Design review of the part built by this model. Coordinates are the model's own, in mm. A direction names the side the tool comes from. Coordinates: 2 decimals unless noted, no trailing zeros. Loops run counter-clockwise (first coordinate to the right, second up) from the corner with the lowest first, then second, coordinate; pieces in that order, holes last.
Q1. Wall thickness on probe 1 along Y at (x, z) = (-2.4, 0.15); probe 2 along X at (y, z) = (-8.5, -0.4); probe 3 along Z at (x, y) = (1.35, -14.25): over which ranges is each line inside the solid? List them lowest first.
Q2. Add section A-A on z = 0. Give the boundary of the cut face in (x, y).
Q3. For P1, Ø3, axis at x = 1, y = -8.5, coming from the -Z side; P2, Ø1, axis at x = 0, y = -5, coming from the +Z side; P3, Ø1.2, axis at x = 0, z = 0, coming from the +Y side, all flat-tipped, find the tip position at first contact; note any pin that passes through.
Q4. Draft analysis for pull direction Z (two halves, no side actions). For faces 3 (the face through (0, -2, 0)), 4 (the face through (0.63, -0.99, -1.08)), 5 (the face through (1.5, -8.92, -0.07)), 6 (the face through (2, -3, 0)), state which applies: released by +Z, released by -Z, zero draft, split by the parting line, or undercut.
Q5. Add section B-B on y = -5.75. Give the boundary of the cut face in (x, z).
Q6. Machinability: for faces 1 (the face through (0.616, -0.987, 1.088)), 2 (the face through (0.596, -1.58, 2.685)), which of the approach directions +Z, -Z, +X, -X, +Y, -Y give a long, thin tool a straight path to every point of the face, cutting with its end or side? Answer none if there is none.
```python
from build123d import *

# Parameters (mm, degrees)
CHAMFER1_SIZE      = 0.25
FILLET1_R          = 0.2
CUT_EXTRUDE1_DEPTH = 2
FILLET2_R          = 0.1


with BuildPart() as part:
    # Sketch1 → Revolve1 (revolve)
    with BuildSketch(Plane.XY):
        Polygon((0, -15), (-1.5, -15), (-1.5, -3), (-2.75, -3), (-2.75, 0), (0, 0), align=None)
    revolve(axis=Axis((0, 0, 0), (0, -1, 0)))

    # Chamfer1
    chamfer1_edges = [part.edges().sort_by_distance(p)[0] for p in [
        (1.5, -3, 0),
        (1.5, -15, 0),
    ]]
    chamfer(chamfer1_edges, length=CHAMFER1_SIZE)

    # Fillet1
    fillet1_edges = [part.edges().sort_by_distance(p)[0] for p in [
        (2.75, 0, 0),
    ]]
    fillet(fillet1_edges, radius=FILLET1_R)

    # Sketch2 → Cut-Extrude1 (cut)
    with BuildSketch(Plane(origin=(0, 0, 0), x_dir=(1, 0, 0), z_dir=(0, 1, 0))):
        Polygon((0, 1.443375673), (-1.25, 0.721687836), (-1.25, -0.721687836), (0, -1.443375673), (1.25, -0.721687836), (1.25, 0.721687836), align=None)
    extrude(amount=-CUT_EXTRUDE1_DEPTH, mode=Mode.SUBTRACT)

    # Fillet2
    fillet2_edges = [part.edges().sort_by_distance(p)[0] for p in [
        (0.625, -2, -1.082531755),
        (1.25, -2, 0),
        (0.625, -2, 1.082531755),
        (-0.625, -2, 1.082531755),
        (-1.25, -2, 0),
        (-0.625, -2, -1.082531755),
        (0.625, 0, -1.082531755),
        (-0.625, 0, -1.082531755),
        (-1.25, 0, 0),
        (-0.625, 0, 1.082531755),
        (0.625, 0, 1.082531755),
        (1.25, 0, 0),
    ]]
    fillet(fillet2_edges, radius=FILLET2_R)


solid = part.part
```
Entries:
1. probe 1: y = -3 to 0
1. probe 2: x = -1.45 to 1.45
1. probe 3: z = -0.65 to 0.65
2. outline: (-2.75, -3) - (-1.75, -3) - (-1.5, -3.25) - (-1.5, -14.75) - (-1.25, -15) - (1.25, -15) - (1.5, -14.75) - (1.5, -3.25) - (1.75, -3) - (2.75, -3) - (2.75, -0.2) arc R0.2 ccw to (2.55, 0) - (1.35, 0) arc R0.1 ccw to (1.25, -0.1) - (1.25, -1.9) arc R0.1 cw to (1.15, -2) - (-1.15, -2) arc R0.1 cw to (-1.25, -1.9) - (-1.25, -0.1) arc R0.1 ccw to (-1.35, 0) - (-2.55, 0) arc R0.2 ccw to (-2.75, -0.2) - close
3. P1: stops at z = -1.5
3. P2: stops at z = 1.5
3. P3: stops at y = -2
4. face 3: undercut
4. face 4: undercut
4. face 5: split by the parting line
4. face 6: zero draft
5. outline: circle Ø3 at (0, 0)
6. face 1: +Y
6. face 2: +Y, -Y
